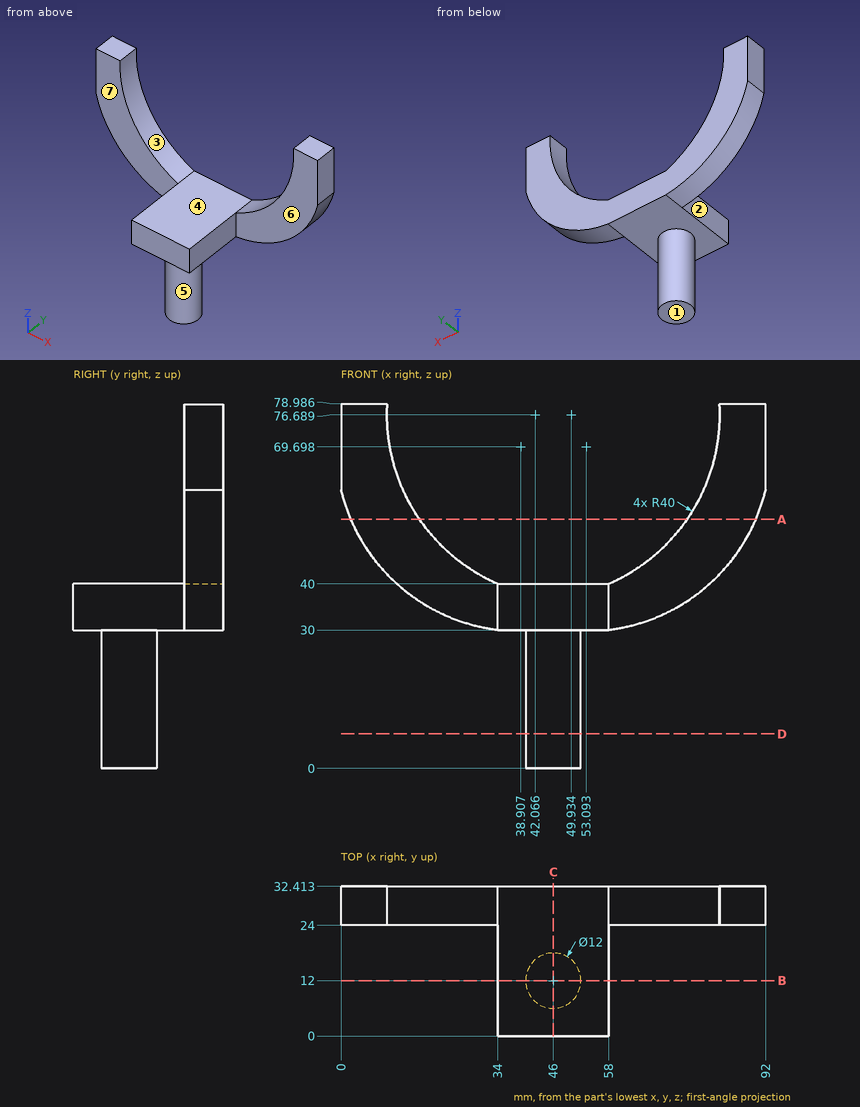
Could you check a few things on this drawing? It's one solid part, dimensions in mm from its lowest x, y, z. A direction names the side the tool comes from. Coordinates: 2 decimals unless noted, no trailing zeros. Order: outer loops, then holes, each group sorted by start corner. A loop starts at its lowest first (then second) coordinate and runs counter-clockwise, first axis right, second up. Notation, with made-up numbers: M 83,83 L 116,83 A16 cw 116,93 Z; hole C -34,-12 d8. An arc over 180 degrees is marked long. Use one line per item in the form item = value. Start each with the question number.
1. Suppose I cut it at D-D on z = 7.5. Write out the boundary of the cut face in (x, y).
2. Please list where these lines run through material, in increasing order: line 1 (Y direction, x = 86.5, z = 49.5); line 2 (Z direction, x = 45, y = 15.5); line 3 (X direction, y = 23.5, z = 31).
3. On a 3-axis mill with a long thin cutter (end or side, diameter ignored), from which of +Z, -Z, +X, -X, +Y, -Y can I reach the whole of each face in a straight line? I mean the marked faces 5, 6 and 7. Say none if no direction works.
4. Suppose I cut it at C-C on x = 46. Write out the boundary of the cut face in (y, z), then the cut area to 3 significant figures.
5. We'd pull the mould along X, two halves only. Please class the marked faces 1, 2, 3 and 4: +X half, -X half, draft (parallel to the pull), parting line (faces both ways), or undercut.
6. For pin 1 (5 mm diameter, centred on y = 12.5, z = 33.5, fed in from +X); pin 2 (1.5 mm diameter, centred on y = 10, z = 41, fed in from +X); pin 3 (12 mm diameter, centred on x = 63, y = 4.5, fed in from +Z); pin 4 (3 mm diameter, centred on y = 16.5, z = 33, fed in from -X), each with a flat end and sliding along its axis, tell me the tip position at first contact or that it passes through.
7. Suppose I cut it at A-A on z = 54. Write out the boundary of the cut face in (x, y) (1 decimal), then the cut area to 3 significant figures.
8. Suppose I cut it at B-B on y = 12. Write out the boundary of the cut face in (x, z).
Geometry says:
q1.outline = C 46,12 d12
q2.line_1 = 24 to 32.41
q2.line_2 = 0 to 40
q2.line_3 = 34 to 58
q3.face_5 = -Z
q3.face_6 = +Z, -Z, +X, -Y
q3.face_7 = +Z, -Z, -X, -Y
q4.outline = M 0,30 L 6,30 L 6,0 L 18,0 L 18,30 L 32.41,30 L 32.41,40 L 0,40 Z
q4.area = 684 mm^2
q5.face_1 = draft
q5.face_2 = -X half
q5.face_3 = undercut
q5.face_4 = undercut
q6.pin_1 = 58
q6.pin_2 = through
q6.pin_3 = 40
q6.pin_4 = 34
q7.outline = M 2.1,24 L 17,24 L 17,32.4 L 2.1,32.4 Z; M 75,24 L 89.9,24 L 89.9,32.4 L 75,32.4 Z
q7.area = 250 mm^2
q8.outline = M 34,30 L 40,30 L 40,0 L 52,0 L 52,30 L 58,30 L 58,40 L 34,40 Z
